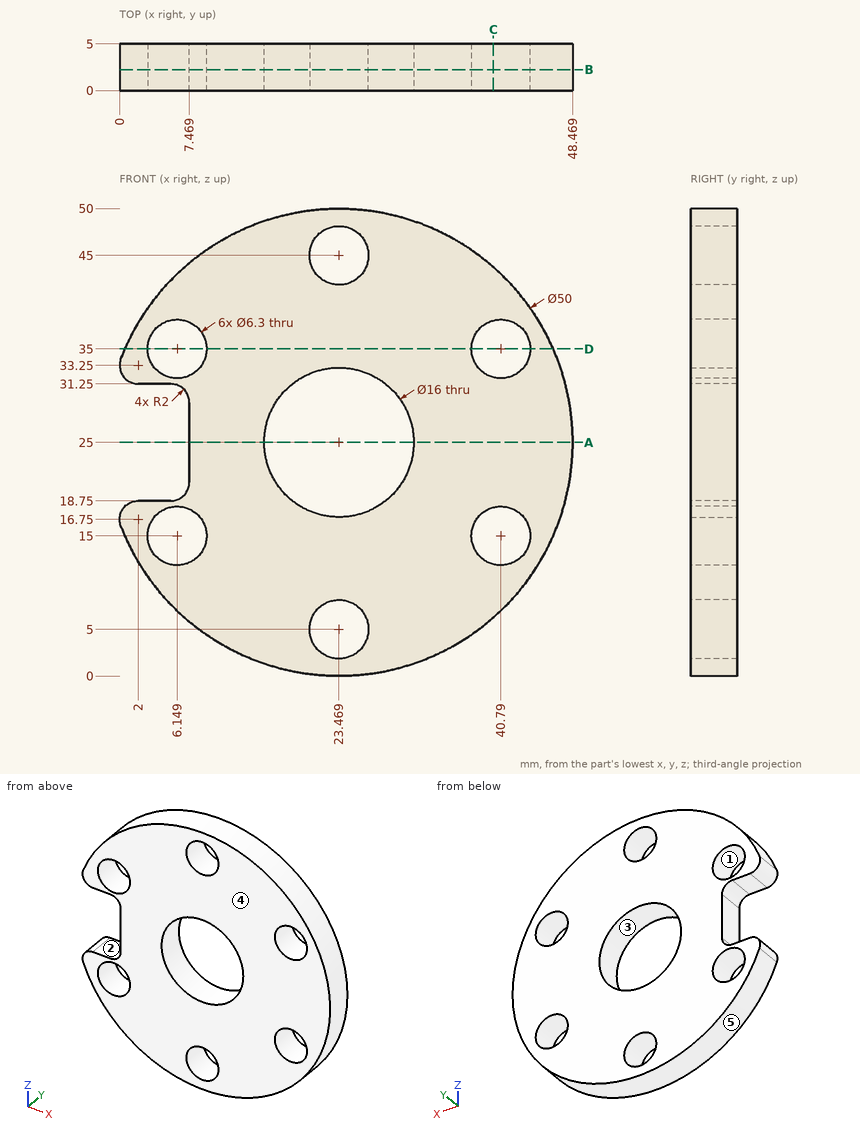
Study the drawing (mm; zero at the part's minimum x, y, z) and answer. A direction names the side the tool comes from. Coordinates: 2 decimals unless noted, no trailing zeros. Write each loop counter-clockwise with the first axis right and the second up, starting at its lowest first coordinate (ties: lowest second). Pieces come first, ordered by that corner, then holes. Notation, with made-up numbers: (88, 11.25) -> (145, 11.25) arc R17 cw to (145, 42.25) -> close; hole circle Ø7 at (84.5, 33). An arc over 180 degrees is marked (long way). Write item = value, one per line.
(1) Which of the six approach directions +Z, -Z, +X, -X, +Y, -Y give full straight-line access (tool end or side, diameter ignored) to the marked faces 1 and 2?
From the geometry:
face_1 = +Y, -Y
face_2 = -X, +Y, -Y
(2) For a pull along X with two mould halves and no side action, classify the marked faces 3, 4 and 5 as +X half, -X half, draft (parallel to the pull), parting line (faces both ways), or undercut.
From the geometry:
face_3 = undercut
face_4 = draft
face_5 = parting line
(3) Straight lines are drawn through the part: L1, parallel to Z at x = 39, y = 4.6; L2, parallel to Z at x = 23, y = 1.35 (1 decimal); L3, parallel to Z at x = 24.5, y = 2.8. For each, find the intervals that lie inside material, in ascending order. Write a range as from..to.
From the geometry:
L1 = 5.41..12.41, 17.59..32.41, 37.59..44.59
L2 = 0..1.9, 8.1..17, 33..41.9, 48.1..50
L3 = 0.02..2.02, 7.98..17.07, 32.93..42.02, 47.98..49.98
(4) Given pin 1 Ø1 at (x, y) = (3.5, 3) entering from +Z; pin 2 Ø3 at (x, y) = (3.5, 2.5) entering from -Z; pin 3 Ø3 at (y, z) = (4.5, 9.5) entering from -X, each flat-ended and moving along its own axis, determine where each tip first touches the part or whether it passes through.
From the geometry:
pin_1 = 40.68
pin_2 = 8.15
pin_3 = 2.76
(5) Section B-B on y = 2.25 is taken. Write down the section's boundary in (x, z), plus the area to 3 significant figures.
From the geometry:
outline = (0.13, 16.03) arc R25 ccw (long way) to (0.13, 33.97) arc R2 ccw to (2, 31.25) -> (5.47, 31.25) arc R2 cw to (7.47, 29.25) -> (7.47, 20.75) arc R2 cw to (5.47, 18.75) -> (2, 18.75) arc R2 ccw to start; hole circle Ø6.3 at (6.15, 15); hole circle Ø6.3 at (6.15, 35); hole circle Ø16 at (23.47, 25); hole circle Ø6.3 at (23.47, 5); hole circle Ø6.3 at (23.47, 45); hole circle Ø6.3 at (40.79, 15); hole circle Ø6.3 at (40.79, 35)
area = 1,460 mm2
(6) Section A-A on z = 25 is taken. Write down the section's boundary in (x, y), plus the area to 3 significant figures.
From the geometry:
outline = (7.47, 0) -> (15.47, 0) -> (15.47, 5) -> (7.47, 5) -> close; (31.47, 0) -> (48.47, 0) -> (48.47, 5) -> (31.47, 5) -> close
area = 125 mm2
(7) Section C-C on x = 40 is taken. Count the separate pieces of the cut face and the enclosed holes in it.
From the geometry:
separate_pieces = 3
enclosed_holes = 0
(8) Section D-D on z = 35 is taken. Write down the section's boundary in (x, y).
From the geometry:
outline = (0.56, 0) -> (3, 0) -> (3, 5) -> (0.56, 5) -> close; (9.3, 0) -> (37.64, 0) -> (37.64, 5) -> (9.3, 5) -> close; (43.94, 0) -> (46.38, 0) -> (46.38, 5) -> (43.94, 5) -> close
